Geometry: final body of the model. Coordinates: model frame, mm. A direction names the side the tool comes from. Coordinates: 2 decimals unless noted, no trailing zeros. Write each loop counter-clockwise with the first axis right and the second up, starting at its lowest first coordinate (ties: lowest second). Pieces come first, ordered by that corner, then holes.
from build123d import *

# Parameters (mm, degrees)
EXTRUDE_1_DEPTH = 8
SKETCH_2_R      = 5
EXTRUDE_2_DEPTH = 50
CHAMFER_1_SIZE  = 2
CHAMFER_1_SIZE2 = 1.154700538


with BuildPart() as part:
    # Эскиз1 → Бобышка-Вытянуть1 (new body)
    with BuildSketch(Plane(origin=(0, 0, 0), x_dir=(1, 0, 0), z_dir=(0, 1, 0))):
        Polygon((8.5, -4.907477288), (8.5, 4.907477288), (0, 9.814954576), (-8.5, 4.907477288), (-8.5, -4.907477288), (0, -9.814954576), align=None)
    extrude(amount=EXTRUDE_1_DEPTH)

    # Эскиз2 → Бобышка-Вытянуть2 (add)
    with BuildSketch(Plane(origin=(0, 8, 0), x_dir=(1, 0, 0), z_dir=(0, 1, 0))):
        Circle(SKETCH_2_R)
    extrude(amount=EXTRUDE_2_DEPTH)

    # Фаска1
    chamfer_1_edges = [part.edges().sort_by_distance(p)[0] for p in [
        (-4.25, 0, 7.361215932),
        (-8.5, 0, 0),
        (-4.25, 0, -7.361215932),
        (4.25, 0, -7.361215932),
        (8.5, 0, 0),
        (4.25, 0, 7.361215932),
    ]]
    chamfer_1_side = [part.faces().sort_by_distance(p)[0] for p in [
        (0, 0, 0),
    ]]
    chamfer(chamfer_1_edges, length=CHAMFER_1_SIZE, length2=CHAMFER_1_SIZE2, reference=chamfer_1_side[0])


solid = part.part
Item 1: Pin query (flat end, axial travel): pin 1 (2 mm diameter, centred on x = 4.5, y = 26.5, fed in from +Z); pin 2 (5 mm diameter, centred on y = 18, z = -0.5, fed in from +X); pin 3 (5 mm diameter, centred on x = -5.5, y = 6.5, fed in from -Z). Return the tip coordinate at first contact, or that it passes through.
Derived:
pin 1: stops at z = 3.57
pin 2: stops at x = 5
pin 3: stops at z = -8.08
Item 2: Section A-A, the plane z = 0. Output: boundary loops of the cut face in (x, y), plus the area to 3 significant figures.
Derived:
outline: (-8.5, 1.15) - (-6.5, 0) - (6.5, 0) - (8.5, 1.15) - (8.5, 8) - (5, 8) - (5, 58) - (-5, 58) - (-5, 8) - (-8.5, 8) - close
area: 634 mm2
Item 3: Material intervals for probe 1 along Y at (x, z) = (-4.5, 2.5); probe 2 along Z at (x, y) = (5, 6.5); probe 3 along Z at (x, y) = (-3.25, 26), sorted ascending.
Derived:
probe 1: y = 0 to 8
probe 2: z = -6.93 to 6.93
probe 3: z = -3.8 to 3.8
Item 4: Section C-C, the plane x = -1.5. Output: boundary loops of the cut face in (y, z).
Derived:
outline: (0, -6.64) - (1.15, -8.95) - (8, -8.95) - (8, -4.77) - (58, -4.77) - (58, 4.77) - (8, 4.77) - (8, 8.95) - (1.15, 8.95) - (0, 6.64) - close
Item 5: Set-up query: faces 1 (the flat face through (4.191, 4.529, 7.396)), 2 (the cylindrical face through (-1.08, 32.65, 4.88)). Return all of +Z, -Z, +X, -X, +Y, -Y with unobstructed straight access to the full face (end or side cutting, diameter ignored); none if empty.
Derived:
face 1: +Z, +X, +Y, -Y
face 2: +Y
Item 6: Section B-B, the plane y = 37. Output: boundary loops of the cut face in (x, z), plus the area to 3 significant figures.
Derived:
outline: circle Ø10 at (0, 0)
area: 78.5 mm2
